from build123d import *

# Parameters (mm, degrees)
F1_R     = 17
F1_R_2   = 15.5
F2_DEPTH = 115
F3_R     = 17
F4_DEPTH = 2
F5_R     = 15.25
F6_DEPTH = 10
F8_R     = 2.25
F9_DEPTH = 70


# Not quite as in the source:
# - a feature of the source that left no trace in its solid (it failed there, or was rolled back) is left out


with BuildPart() as f2:
    # F1 (on offset) → F2 (new body)
    with BuildSketch(Plane.XY.offset(107)):
        Circle(F1_R)
        Circle(F1_R_2, mode=Mode.SUBTRACT)
    extrude(amount=F2_DEPTH)

    # F3 (on offset) → F4 (join)
    with BuildSketch(Plane.XY.offset(107)):
        Circle(F3_R)
    extrude(amount=F4_DEPTH)

    # F5 (on face) → F6 (join)
    with BuildSketch(Plane(origin=(0, 0, 107), x_dir=(1, 0, 0), z_dir=(0, 0, -1))):
        Circle(F5_R)
    extrude(amount=F6_DEPTH)

    # F8 (on offset) → F9 (join)
    with BuildSketch(Plane.XY.offset(127)):
        with BuildLine():
            Line((20.2600458013, 3.5), (16.2600458013, 3.5))
            Line((16.2600458013, 3.5), (16.2600458013, -3.5))
            Line((16.2600458013, -3.5), (20.2600458013, -3.5))
            ThreePointArc((20.2600458013, -3.5), (22.3813661449, -2.6213203436), (23.2600458013, -0.5))
            Line((23.2600458013, -0.5), (23.2600458013, 0.5))
            ThreePointArc((23.2600458013, 0.5), (22.3813661449, 2.6213203436), (20.2600458013, 3.5))
        make_face()
        with Locations((19.7600458013, 0)):
            Circle(F8_R, mode=Mode.SUBTRACT)
    extrude(amount=F9_DEPTH)


solid = f2.part
Part model, mm, in its own coordinate system. A direction names the side the tool comes from. Coordinates: 2 decimals unless noted, no trailing zeros. Order: outer loops, then holes, each group sorted by start corner. A loop starts at its lowest first (then second) coordinate and runs counter-clockwise, first axis right, second up.
(1) Pin check, flat tips, straight feed: pin 1 Ø10 at (y, z) = (10, 179.5) entering from -X; pin 2 Ø5 at (x, y) = (19.76, 0) entering from +Z; pin 3 Ø1.8 at (x, z) = (18, 169.5) entering from +Y. Stop position of each tip, or through.
Check sheet entries:
pin 1: stops at x = -16.25
pin 2: stops at z = 197
pin 3: stops at y = 3.5
(2) Slice it at C-C, the plane z = 204.5. Write the cut outline in (x, y), and give its area (3 significant figures).
Check sheet entries:
outline: circle Ø34 at (0, 0); hole circle Ø31 at (0, 0)
area: 153 mm2
(3) Tool access for faces 1 (the face through (18, -3.5, 162)), 2 (the face through (18, 3.5, 162)), 3 (the face through (-13, -9, 107)): list every direction of +Z, -Z, +X, -X, +Y, -Y with a clear straight run to the whole face (end or side of a thin tool).
Check sheet entries:
face 1: +Z, -Z, +X, -Y
face 2: +Z, -Z, +X, +Y
face 3: -Z
(4) Probe L1, parallel to Y at x = 0, z = 188; L2, parallel to Z at x = 10, y = 13; L3, parallel to Z at x = -7, y = 12.5. List the from-to ranges inside material, lowest first.
Check sheet entries:
L1: y = -17 to -15.5, 15.5 to 17
L2: z = 107 to 222
L3: z = 97 to 109
(5) Slice it at D-D, the plane y = -9. Write the cut outline in (x, z), and give its area (3 significant figures).
Check sheet entries:
outline: (-14.42, 107) - (-12.31, 107) - (-12.31, 97) - (12.31, 97) - (12.31, 107) - (14.42, 107) - (14.42, 222) - (12.62, 222) - (12.62, 109) - (-12.62, 109) - (-12.62, 222) - (-14.42, 222) - close
area: 711 mm2
(6) Pull direction Y, two halves, no side cores. Call faces 4 (the face through (19.9, 2.4, 197)), 5 (the face through (18.1, 1.52, 161.51)), 6 (the face through (22.4, -2.6, 161.5)): pulls with the +Y half, pulls with the -Y half, needs draft (parallel to the pull), parting line crosses it, or undercut.
Check sheet entries:
face 4: needs draft
face 5: undercut
face 6: pulls with the -Y half
(7) Slice it at B-B, the plane x = 0. Write the cut outline in (y, z), and give its area (3 significant figures).
Check sheet entries:
outline: (-17, 107) - (-15.25, 107) - (-15.25, 97) - (15.25, 97) - (15.25, 107) - (17, 107) - (17, 222) - (15.5, 222) - (15.5, 109) - (-15.5, 109) - (-15.5, 222) - (-17, 222) - close
area: 712 mm2
(8) Slice it at A-A, the plane z = 155. Write the cut outline in (x, y), and give its area (3 significant figures).
Check sheet entries:
outline: (16.64, -3.5) - (20.26, -3.5) arc R3 ccw to (23.26, -0.5) - (23.26, 0.5) arc R3 ccw to (20.26, 3.5) - (16.64, 3.5) arc R17 ccw (long way) to start; hole circle Ø31 at (0, 0); hole circle Ø4.5 at (19.76, 0)
area: 178 mm2
